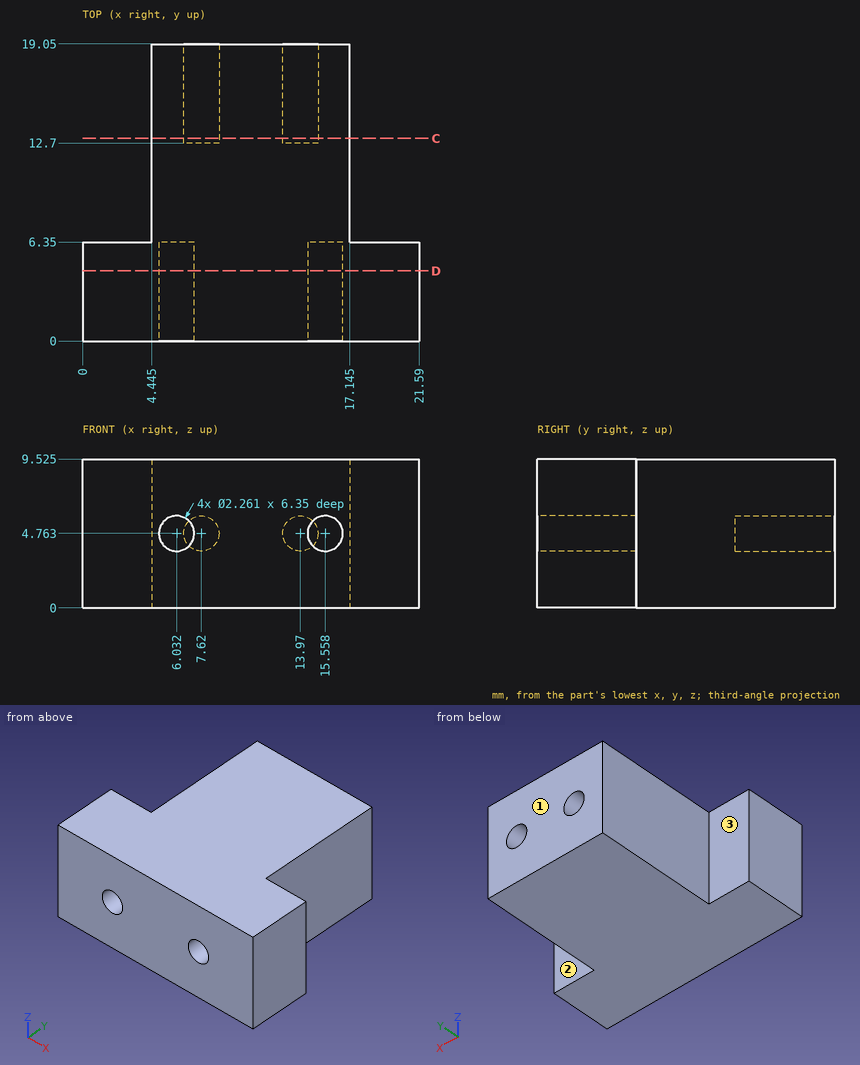
Answer from the drawing. Dimensions are ordinates in mm from the lowest x, y and z of the part. A direction names the side the tool comes from. Round coordinates to 2 decimals unless told otherwise and drop trailing zeros. Order: outer loops, then holes, each group sorted by start corner. A loop starts at its lowest first (then second) coordinate and runs counter-clockwise, first axis right, second up. Notation, with made-up numbers: (63, 3.25) -> (79, 3.25) arc R29 cw to (79, 24.25) -> close; hole circle Ø6 at (26.5, 87.25). An arc over 180 degrees is marked (long way). Answer as CSV lines item,"result".
Q1. Which of the six approach directions +Z, -Z, +X, -X, +Y, -Y give full straight-line access (tool end or side, diameter ignored) to the marked faces 1, 2 and 3?
Computed values:
face 1,"+Z, -Z, +X, -X, +Y"
face 2,"+Z, -Z, +X, +Y"
face 3,"+Z, -Z, -X, +Y"
Q2. Consider line 1 (Z direction, x = 7.62, y = 16.25) (1 decimal); line 2 (X direction, y = 13, z = 5.75) (1 decimal); line 3 (X direction, y = 1.75, z = 4.5). Determine where each line is inside the solid, lowest interval first. Write a range as from..to.
Computed values:
line 1,"z = 0..3.6, 5.9..9.5"
line 2,"x = 4.4..7.1, 8.2..13.4, 14.5..17.1"
line 3,"x = 0..4.93, 7.13..14.46, 16.66..21.59"
Q3. A cutting plane is placed at D-D on y = 4.5. Determine the outline of the cut face in (x, z) (1 decimal), plus the area to 3 significant figures.
Computed values:
outline,"(0, 0) -> (21.6, 0) -> (21.6, 9.5) -> (0, 9.5) -> close; hole circle Ø2.3 at (6, 4.8); hole circle Ø2.3 at (15.6, 4.8)"
area,"198 mm^2"
Q4. Given pin 1 (2.5 mm diameter, centred on x = 13.97, z = 4.76, fed in from -Y); pin 2 (2 mm diameter, centred on x = 3, z = 5, fed in from +Y); pin 3 (3 mm diameter, centred on y = 17, z = 3.5, fed in from +X) (1 decimal); pin 4 (2 mm diameter, centred on x = 15.56, z = 4.76, fed in from -Y), each flat-ended and moving along its own axis, determine where each tip first touches the part or whether it passes through.
Computed values:
pin 1,"stops at y = 0"
pin 2,"stops at y = 6.35"
pin 3,"stops at x = 17.1"
pin 4,"stops at y = 6.35"
Q5. A cutting plane is placed at C-C on y = 13. Give the number of separate pieces and of enclosed holes in the cut face, plus the area to 3 significant figures.
Computed values:
separate pieces,"1"
enclosed holes,"2"
area,"113 mm^2"
